Source: CAD feature listing. Evaluate the final solid. Frame: model axes, mm. Face numbers are marked on the shaded views. Give positions to 0.01 mm unless a question says otherwise; leave off trailing zeros. Loops run counter-clockwise (first coordinate to the right, second up) from the corner with the lowest first, then second, coordinate; pieces in that order, holes last. Notation, with made-up numbers: M 6,-24 L 19,-24 A32 cw 19,9 Z; hole C 54.25,39.25 d7. An arc over 180 degrees is marked long. Answer in a Markdown table with one row per item.
```python
from build123d import *

# Parameters (mm, degrees)
SKETCH1_W               = 78
SKETCH1_H               = 46
BOSS_EXTRUDE1_DEPTH     = 4.2
SKETCH2_W               = 8.5
SKETCH2_H               = 2
CUT_EXTRUDE1_DEPTH      = 20.65
CUT_EXTRUDE2_DEPTH      = 7.4
BOSS_EXTRUDE3_DEPTH     = 23
LPATTERN1_COUNT         = 6
LPATTERN1_PITCH         = 11
MIRROR3_COPY_1_SKETCH_W = 8.5
MIRROR3_COPY_1_SKETCH_H = 2
MIRROR3_COPY_1_DEPTH    = 20.65
MIRROR3_COPY_2_SKETCH_W = 8.5
MIRROR3_COPY_2_SKETCH_H = 2
MIRROR3_COPY_2_DEPTH    = 20.65
MIRROR3_COPY_3_SKETCH_W = 8.5
MIRROR3_COPY_3_SKETCH_H = 2
MIRROR3_COPY_3_DEPTH    = 20.65
MIRROR3_COPY_4_SKETCH_W = 8.5
MIRROR3_COPY_4_SKETCH_H = 2
MIRROR3_COPY_4_DEPTH    = 20.65
MIRROR3_COPY_5_SKETCH_W = 8.5
MIRROR3_COPY_5_SKETCH_H = 2
MIRROR3_COPY_5_DEPTH    = 20.65
MIRROR3_COPY_6_DEPTH    = 7.4
MIRROR3_COPY_7_DEPTH    = 7.4
MIRROR3_COPY_8_DEPTH    = 7.4
MIRROR3_COPY_9_DEPTH    = 7.4
MIRROR3_COPY_10_DEPTH   = 7.4
MIRROR3_COPY_11_DEPTH   = 23
MIRROR3_COPY_12_DEPTH   = 23
MIRROR3_COPY_13_DEPTH   = 23
MIRROR3_COPY_14_DEPTH   = 23
MIRROR3_COPY_15_DEPTH   = 23
SKETCH6_W               = 8.5
SKETCH6_H               = 20.65
BOSS_EXTRUDE2_DEPTH     = 8.4
SKETCH4_R               = 1.5
CUT_EXTRUDE3_DEPTH      = 5
SKETCH7_R               = 1.1
CUT_EXTRUDE4_DEPTH      = 10
SKETCH9_W               = 4.15
SKETCH9_H               = 1.8
CUT_EXTRUDE5_DEPTH      = 9.4
SKETCH10_W              = 4.15
SKETCH10_H              = 1.8
CUT_EXTRUDE6_DEPTH      = 9.4
SKETCH11_R              = 1.1
CUT_EXTRUDE7_DEPTH      = 8
LPATTERN2_COUNT         = 2
LPATTERN2_PITCH         = 22
CUT_EXTRUDE8_DEPTH      = 19.05
CUT_EXTRUDE9_DEPTH      = 19.05
LPATTERN3_COUNT         = 3
LPATTERN3_PITCH         = 22
LPATTERN4_COUNT         = 3
LPATTERN4_PITCH         = 22
FILLET1_R               = 0.25


with BuildPart() as part:
    # Sketch1 → Boss-Extrude1 (new body, symmetric)
    with BuildSketch(Plane(origin=(0, 0, 0), x_dir=(1, 0, 0), z_dir=(0, 1, 0))):
        Rectangle(SKETCH1_W, SKETCH1_H)
    extrude(amount=BOSS_EXTRUDE1_DEPTH, both=True)

    # Sketch2 → Cut-Extrude1 (cut)
    with BuildSketch(Plane(origin=(0, 0, -23), x_dir=(-1, 0, 0), z_dir=(0, 0, -1))):
        with Locations((-27.5, 3.2)):
            Rectangle(SKETCH2_W, SKETCH2_H)
    cut_extrude1 = extrude(amount=-CUT_EXTRUDE1_DEPTH, mode=Mode.SUBTRACT)

    # Sketch3 → Cut-Extrude2 (cut, through all)
    with BuildSketch(Plane(origin=(0, 2.2, 0), x_dir=(1, 0, 0), z_dir=(0, 1, 0))):
        Polygon((24.25, 21.3), (23.25, 20.3), (23.25, 4.95), (24.25, 3.95), (30, 3.95), (30, 21.3), align=None)
        Polygon((30, 23), (23.25, 23), (23.25, 20.3), (24.25, 21.3), (30, 21.3), align=None)
    cut_extrude2 = extrude(amount=-CUT_EXTRUDE2_DEPTH, mode=Mode.SUBTRACT)

    # Sketch15 → Boss-Extrude3 (add)
    with BuildSketch(Plane.XY):
        Polygon((30, -4.2), (26.75, -4.2), (30, -0.95), align=None)
    boss_extrude3 = extrude(amount=-BOSS_EXTRUDE3_DEPTH)

    # LPattern1: Cut-Extrude1, Cut-Extrude2, Boss-Extrude3 ×6
    with Locations(*[(-i * LPATTERN1_PITCH, 0, 0) for i in range(1, LPATTERN1_COUNT)]):
        add(cut_extrude1, mode=Mode.SUBTRACT)
        add(cut_extrude2, mode=Mode.SUBTRACT)
        add(boss_extrude3)

    # Mirror3: Cut-Extrude1, Cut-Extrude2, Boss-Extrude3 across plane
    add(cut_extrude1.mirror(Plane.XY), mode=Mode.SUBTRACT)
    add(cut_extrude2.mirror(Plane.XY), mode=Mode.SUBTRACT)
    add(boss_extrude3.mirror(Plane.XY))

    # Mirror3 copy 1 sketch → Mirror3 copy 1 (cut)
    with BuildSketch(Plane(origin=(-11, 0, 23), x_dir=(-1, 0, 0), z_dir=(0, 0, 1))):
        with Locations((-27.5, -3.2)):
            Rectangle(MIRROR3_COPY_1_SKETCH_W, MIRROR3_COPY_1_SKETCH_H)
    extrude(amount=-MIRROR3_COPY_1_DEPTH, mode=Mode.SUBTRACT)

    # Mirror3 copy 2 sketch → Mirror3 copy 2 (cut)
    with BuildSketch(Plane(origin=(-22, 0, 23), x_dir=(-1, 0, 0), z_dir=(0, 0, 1))):
        with Locations((-27.5, -3.2)):
            Rectangle(MIRROR3_COPY_2_SKETCH_W, MIRROR3_COPY_2_SKETCH_H)
    extrude(amount=-MIRROR3_COPY_2_DEPTH, mode=Mode.SUBTRACT)

    # Mirror3 copy 3 sketch → Mirror3 copy 3 (cut)
    with BuildSketch(Plane(origin=(-33, 0, 23), x_dir=(-1, 0, 0), z_dir=(0, 0, 1))):
        with Locations((-27.5, -3.2)):
            Rectangle(MIRROR3_COPY_3_SKETCH_W, MIRROR3_COPY_3_SKETCH_H)
    extrude(amount=-MIRROR3_COPY_3_DEPTH, mode=Mode.SUBTRACT)

    # Mirror3 copy 4 sketch → Mirror3 copy 4 (cut)
    with BuildSketch(Plane(origin=(-44, 0, 23), x_dir=(-1, 0, 0), z_dir=(0, 0, 1))):
        with Locations((-27.5, -3.2)):
            Rectangle(MIRROR3_COPY_4_SKETCH_W, MIRROR3_COPY_4_SKETCH_H)
    extrude(amount=-MIRROR3_COPY_4_DEPTH, mode=Mode.SUBTRACT)

    # Mirror3 copy 5 sketch → Mirror3 copy 5 (cut)
    with BuildSketch(Plane(origin=(-55, 0, 23), x_dir=(-1, 0, 0), z_dir=(0, 0, 1))):
        with Locations((-27.5, -3.2)):
            Rectangle(MIRROR3_COPY_5_SKETCH_W, MIRROR3_COPY_5_SKETCH_H)
    extrude(amount=-MIRROR3_COPY_5_DEPTH, mode=Mode.SUBTRACT)

    # Mirror3 copy 6 sketch → Mirror3 copy 6 (cut, through all)
    with BuildSketch(Plane(origin=(-11, 2.2, 0), x_dir=(1, 0, 0), z_dir=(0, 1, 0))):
        Polygon((24.25, -21.3), (23.25, -20.3), (23.25, -4.95), (24.25, -3.95), (30, -3.95), (30, -21.3), align=None)
        Polygon((30, -23), (23.25, -23), (23.25, -20.3), (24.25, -21.3), (30, -21.3), align=None)
    extrude(amount=-MIRROR3_COPY_6_DEPTH, mode=Mode.SUBTRACT)

    # Mirror3 copy 7 sketch → Mirror3 copy 7 (cut, through all)
    with BuildSketch(Plane(origin=(-22, 2.2, 0), x_dir=(1, 0, 0), z_dir=(0, 1, 0))):
        Polygon((24.25, -21.3), (23.25, -20.3), (23.25, -4.95), (24.25, -3.95), (30, -3.95), (30, -21.3), align=None)
        Polygon((30, -23), (23.25, -23), (23.25, -20.3), (24.25, -21.3), (30, -21.3), align=None)
    extrude(amount=-MIRROR3_COPY_7_DEPTH, mode=Mode.SUBTRACT)

    # Mirror3 copy 8 sketch → Mirror3 copy 8 (cut, through all)
    with BuildSketch(Plane(origin=(-33, 2.2, 0), x_dir=(1, 0, 0), z_dir=(0, 1, 0))):
        Polygon((24.25, -21.3), (23.25, -20.3), (23.25, -4.95), (24.25, -3.95), (30, -3.95), (30, -21.3), align=None)
        Polygon((30, -23), (23.25, -23), (23.25, -20.3), (24.25, -21.3), (30, -21.3), align=None)
    extrude(amount=-MIRROR3_COPY_8_DEPTH, mode=Mode.SUBTRACT)

    # Mirror3 copy 9 sketch → Mirror3 copy 9 (cut, through all)
    with BuildSketch(Plane(origin=(-44, 2.2, 0), x_dir=(1, 0, 0), z_dir=(0, 1, 0))):
        Polygon((24.25, -21.3), (23.25, -20.3), (23.25, -4.95), (24.25, -3.95), (30, -3.95), (30, -21.3), align=None)
        Polygon((30, -23), (23.25, -23), (23.25, -20.3), (24.25, -21.3), (30, -21.3), align=None)
    extrude(amount=-MIRROR3_COPY_9_DEPTH, mode=Mode.SUBTRACT)

    # Mirror3 copy 10 sketch → Mirror3 copy 10 (cut, through all)
    with BuildSketch(Plane(origin=(-55, 2.2, 0), x_dir=(1, 0, 0), z_dir=(0, 1, 0))):
        Polygon((24.25, -21.3), (23.25, -20.3), (23.25, -4.95), (24.25, -3.95), (30, -3.95), (30, -21.3), align=None)
        Polygon((30, -23), (23.25, -23), (23.25, -20.3), (24.25, -21.3), (30, -21.3), align=None)
    extrude(amount=-MIRROR3_COPY_10_DEPTH, mode=Mode.SUBTRACT)

    # Mirror3 copy 11 sketch → Mirror3 copy 11 (add)
    with BuildSketch(Plane(origin=(-11, 0, 0), x_dir=(1, 0, 0), z_dir=(0, 0, -1))):
        Polygon((30, 4.2), (26.75, 4.2), (30, 0.95), align=None)
    extrude(amount=-MIRROR3_COPY_11_DEPTH)

    # Mirror3 copy 12 sketch → Mirror3 copy 12 (add)
    with BuildSketch(Plane(origin=(-22, 0, 0), x_dir=(1, 0, 0), z_dir=(0, 0, -1))):
        Polygon((30, 4.2), (26.75, 4.2), (30, 0.95), align=None)
    extrude(amount=-MIRROR3_COPY_12_DEPTH)

    # Mirror3 copy 13 sketch → Mirror3 copy 13 (add)
    with BuildSketch(Plane(origin=(-33, 0, 0), x_dir=(1, 0, 0), z_dir=(0, 0, -1))):
        Polygon((30, 4.2), (26.75, 4.2), (30, 0.95), align=None)
    extrude(amount=-MIRROR3_COPY_13_DEPTH)

    # Mirror3 copy 14 sketch → Mirror3 copy 14 (add)
    with BuildSketch(Plane(origin=(-44, 0, 0), x_dir=(1, 0, 0), z_dir=(0, 0, -1))):
        Polygon((30, 4.2), (26.75, 4.2), (30, 0.95), align=None)
    extrude(amount=-MIRROR3_COPY_14_DEPTH)

    # Mirror3 copy 15 sketch → Mirror3 copy 15 (add)
    with BuildSketch(Plane(origin=(-55, 0, 0), x_dir=(1, 0, 0), z_dir=(0, 0, -1))):
        Polygon((30, 4.2), (26.75, 4.2), (30, 0.95), align=None)
    extrude(amount=-MIRROR3_COPY_15_DEPTH)

    # Sketch6 → Boss-Extrude2 (add)
    with BuildSketch(Plane(origin=(0, 4.2, 0), x_dir=(1, 0, 0), z_dir=(0, 1, 0))):
        with Locations((-16.5, 12.675)):
            Rectangle(SKETCH6_W, SKETCH6_H)
        with Locations((5.5, 12.675)):
            Rectangle(SKETCH6_W, SKETCH6_H)
        with Locations((27.5, 12.675)):
            Rectangle(SKETCH6_W, SKETCH6_H)
        with Locations((-27.5, -12.675)):
            Rectangle(SKETCH6_W, SKETCH6_H)
        with Locations((-5.5, -12.675)):
            Rectangle(SKETCH6_W, SKETCH6_H)
        with Locations((16.5, -12.675)):
            Rectangle(SKETCH6_W, SKETCH6_H)
    extrude(amount=-BOSS_EXTRUDE2_DEPTH)

    # Sketch4 → Cut-Extrude3 (cut)
    with BuildSketch(Plane.ZY.offset(39)):
        with Locations((-20, -2.2)):
            Circle(SKETCH4_R)
        with Locations((20, -2.2)):
            Circle(SKETCH4_R)
    cut_extrude3 = extrude(amount=-CUT_EXTRUDE3_DEPTH, mode=Mode.SUBTRACT)

    # Mirror1: Cut-Extrude3 across plane
    add(cut_extrude3.mirror(Plane(origin=(0, 0, 0), x_dir=(0, 0, 1), z_dir=(1, 0, 0))), mode=Mode.SUBTRACT)

    # Sketch7 → Cut-Extrude4 (cut)
    with BuildSketch(Plane.XY.offset(23)):
        with Locations((-5.5, 0)):
            Circle(SKETCH7_R)
        with Locations((16.5, 0)):
            Circle(SKETCH7_R)
    extrude(amount=-CUT_EXTRUDE4_DEPTH, mode=Mode.SUBTRACT)

    # Sketch9 → Cut-Extrude5 (cut, through all)
    with BuildSketch(Plane(origin=(0, 4.2, 0), x_dir=(1, 0, 0), z_dir=(0, 1, 0))):
        with Locations((-5.5, -18)):
            Rectangle(SKETCH9_W, SKETCH9_H)
        Polygon((18.575, -18.9), (14.425, -17.1), (14.425, -18.9), align=None)
        Polygon((18.575, -17.1), (14.425, -17.1), (18.575, -18.9), align=None)
    extrude(amount=-CUT_EXTRUDE5_DEPTH, mode=Mode.SUBTRACT)

    # Sketch10 → Cut-Extrude6 (cut, through all)
    with BuildSketch(Plane(origin=(0, 4.2, 0), x_dir=(1, 0, 0), z_dir=(0, 1, 0))):
        with Locations((-16.5, 18)):
            Rectangle(SKETCH10_W, SKETCH10_H)
    cut_extrude6 = extrude(amount=-CUT_EXTRUDE6_DEPTH, mode=Mode.SUBTRACT)

    # Sketch11 → Cut-Extrude7 (cut)
    with BuildSketch(Plane(origin=(0, 0, -23), x_dir=(-1, 0, 0), z_dir=(0, 0, -1))):
        with Locations((16.5, 0)):
            Circle(SKETCH11_R)
    cut_extrude7 = extrude(amount=-CUT_EXTRUDE7_DEPTH, mode=Mode.SUBTRACT)

    # LPattern2: Cut-Extrude6, Cut-Extrude7 ×2
    with Locations(*[(i * LPATTERN2_PITCH, 0, 0) for i in range(1, LPATTERN2_COUNT)]):
        add(cut_extrude6, mode=Mode.SUBTRACT)
        add(cut_extrude7, mode=Mode.SUBTRACT)

    # Sketch12 → Cut-Extrude8 (cut)
    with BuildSketch(Plane(origin=(0, 0, -23), x_dir=(-1, 0, 0), z_dir=(0, 0, -1))):
        Polygon((-20.75, 2.2), (-22.35, 0.6), (-19, 0.6), (-19, 2.2), align=None)
    cut_extrude8 = extrude(amount=-CUT_EXTRUDE8_DEPTH, mode=Mode.SUBTRACT)

    # Sketch13 → Cut-Extrude9 (cut)
    with BuildSketch(Plane.XY.offset(23)):
        Polygon((31.75, 2.2), (33.35, 0.6), (30, 0.6), (30, 2.2), align=None)
    cut_extrude9 = extrude(amount=-CUT_EXTRUDE9_DEPTH, mode=Mode.SUBTRACT)

    # LPattern3: Cut-Extrude8 ×3
    with Locations(*[(-i * LPATTERN3_PITCH, 0, 0) for i in range(1, LPATTERN3_COUNT)]):
        add(cut_extrude8, mode=Mode.SUBTRACT)

    # LPattern4: Cut-Extrude9 ×3
    with Locations(*[(-i * LPATTERN4_PITCH, 0, 0) for i in range(1, LPATTERN4_COUNT)]):
        add(cut_extrude9, mode=Mode.SUBTRACT)

    # Fillet1
    fillet1_edges = [part.edges().sort_by_distance(p)[0] for p in [
        (22.35, 0.6, -13.475),
        (33.35, 0.6, 13.475),
        (0.35, 0.6, -13.475),
        (-21.65, 0.6, -13.475),
        (11.35, 0.6, 13.475),
        (-10.65, 0.6, 13.475),
    ]]
    fillet(fillet1_edges, radius=FILLET1_R)


with BuildPart() as body_2:
    # Split1: the piece on the far side of the plane
    add(part.part)
    split(bisect_by=Plane(origin=(-6.5, 0, 0), x_dir=(0, 0, 1), z_dir=(1, 0, 0)), keep=Keep.BOTTOM)


with BuildPart() as part_1:
    add(part.part)

    # Split1
    split(bisect_by=Plane(origin=(-6.5, 0, 0), x_dir=(0, 0, 1), z_dir=(1, 0, 0)), keep=Keep.TOP)


solid = body_2.part
```
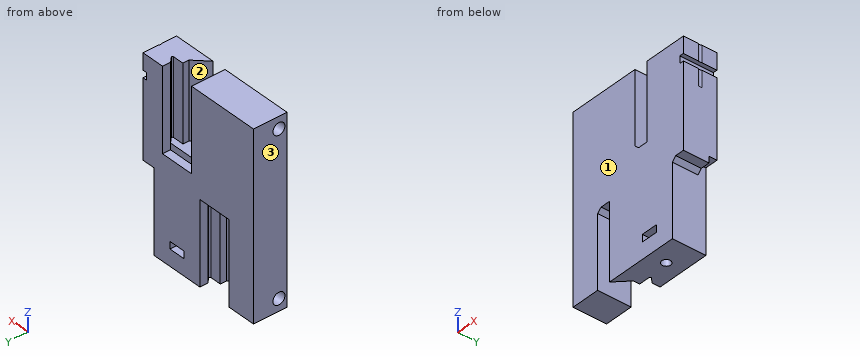
1) Section B-B, the plane x = -16.5. Return loops of the section in (y, z).
Reply:
| item | result |
|---|---|
| outline | M -4.2,-23 L -1.1,-23 L -1.1,-18.9 L -4.2,-18.9 Z; M -4.2,-17.1 L -1.1,-17.1 L -1.1,-15 L 1.1,-15 L 1.1,-17.1 L 4.2,-17.1 L 4.2,2.35 L 2.2,2.35 L 2.2,3.95 L -3.45,3.95 L -3.45,23 L -4.2,23 Z; M 1.1,-23 L 4.2,-23 L 4.2,-18.9 L 1.1,-18.9 Z |
2) Section D-D, the plane y = 3.25. Return loops of the section in (x, z) (3 decimals), then the cut area to 3 significant figures.
Reply:
| item | result |
|---|---|
| outline | M -39,-23 L -31.75,-23 L -31.75,-2.35 L -23.25,-2.35 L -23.25,-23 L -9.75,-23 L -9.75,-2.35 L -6.5,-2.35 L -6.5,17.1 L -7.575,17.1 L -7.575,18.9 L -6.5,18.9 L -6.5,23 L -12.25,23 L -12.25,2.35 L -20.75,2.35 L -20.75,23 L -39,23 Z; hole M -18.575,-18.9 L -14.425,-18.9 L -14.425,-17.1 L -18.575,-17.1 Z |
| area | 1,070 mm² |
3) Pin query (flat end, axial travel): pin 1 Ø4 at (y, z) = (0, -13.5) entering from +X; pin 2 Ø0.9 at (x, y) = (-7, -1) entering from -Z; pin 3 Ø2 at (x, y) = (-26, 3.5) entering from -Z. Return the tip coordinate at first contact, or that it passes through.
Reply:
| item | result |
|---|---|
| pin 1 | stops at x = -9.75 |
| pin 2 | stops at z = -3.95 |
| pin 3 | stops at z = -2.35 |
4) Material intervals for L1, parallel to Y at x = -37, z = 20; L2, parallel to Z at x = -18.5, y = -1.75; L3, parallel to X at y = 3.75, z = 11.5, sorted ascending.
Reply:
| item | result |
|---|---|
| L1 | y = -4.2 to -3.7, -0.7 to 4.2 |
| L2 | z = -23 to -18.9, -17.1 to 3.95 |
| L3 | x = -39 to -20.75, -12.25 to -6.5 |
5) Section C-C, the plane z = 20. Return loops of the section in (x, y), then the cut area to 3 significant figures.
Reply:
| item | result |
|---|---|
| outline | M -39,-4.2 L -20.75,-4.2 L -20.75,4.2 L -39,4.2 L -39,-0.7 L -34,-0.7 L -34,-3.7 L -39,-3.7 Z; M -17.25,-4.2 L -6.5,-4.2 L -6.5,-0.46 A1.1 cw -6.5,0.46 L -6.5,4.2 L -12.25,4.2 L -12.25,2.2 L -11.08,1.03 A0.25 cw -11.25,0.6 L -14,0.6 L -14,-0.95 Z |
| area | 199 mm² |
6) Pull-direction query (X, two-part tool) for the marked faces 1, 2 and 3; classes: released by +X, released by -X, zero draft, split by the parting line, or undercut.
Reply:
| item | result |
|---|---|
| face 1 | zero draft |
| face 2 | undercut |
| face 3 | released by -X |
7) Section A-A, the plane z = -20. Return loops of the section in (x, y).
Reply:
| item | result |
|---|---|
| outline | M -39,-4.2 L -31.75,-4.2 L -31.75,4.2 L -39,4.2 L -39,-0.7 L -34,-0.7 L -34,-3.7 L -39,-3.7 Z; M -28.25,-4.2 L -9.75,-4.2 L -9.75,4.2 L -23.25,4.2 L -23.25,2.2 L -22.08,1.03 A0.25 cw -22.25,0.6 L -25,0.6 L -25,-0.95 Z; hole C -16.5,0 d2.2 |
